Source: CAD feature listing. Evaluate the final solid. Frame: model axes, mm. A direction names the side the tool comes from. Coordinates: 2 decimals unless noted, no trailing zeros. Order: outer loops, then holes, each group sorted by start corner. A loop starts at its lowest first (then second) coordinate and runs counter-clockwise, first axis right, second up.
Autodesk Inventor part; units mm, degrees
ref_plane "YZ Plane" through (0, 0, 0) normal (1, 0, 0) x (0, 1, 0)
ref_plane "XZ Plane" through (0, 0, 0) normal (0, 1, 0) x (-1, 0, 0)
ref_plane "XY Plane" through (0, 0, 0) normal (0, 0, 1) x (1, 0, 0)
sketch "Sketch1" plane through (0, 0, 0) normal (0, 1, 0) x (-1, 0, 0)
  line L0 (0, 0) -> (-38.1, 0)
  line L1 (-38.1, 0) -> (-38.1, -38.1)
  line L2 (-38.1, -38.1) -> (0, -38.1)
  line L3 (0, -38.1) -> (0, 0)
  dimension "d0" = 38.1
  dimension "d1" = 38.1
extrude "Extrusion1" add sketch "Sketch1" along normal blind 25.4
fillet "Fillet1" radius 19.05 1 edges at (0, 12.7, 0)
sketch "Sketch2" plane through (0, 25.4, 0) normal (0, 1, 0) x (1, 0, 0)
  arc A0 (0, 19.05) -> (19.05, 0) centre (19.05, 19.05) ccw
  line L0 (0, 38.1) -> (0, 19.05)
  line L1 (38.1, 38.1) -> (0, 38.1)
  line L2 (38.1, 0) -> (38.1, 38.1)
  line L3 (19.05, 0) -> (38.1, 0)
  arc A1 (-2.8591, 19.05) -> (19.05, -2.8591) centre (19.05, 19.05) ccw
  line L4 (-2.8591, 19.05) -> (-2.8591, 40.9591)
  line L5 (-2.8591, 40.9591) -> (40.9591, 40.9591)
  line L6 (40.9591, 40.9591) -> (40.9591, -2.8591)
  line L7 (40.9591, -2.8591) -> (19.05, -2.8591)
  line L8 (0, 38.1) -> (0, 40.9591)
  line L9 (38.1, 0) -> (40.9591, 0)
  point P0 (0, 0)
extrude "Extrusion2" add sketch "Sketch2" along normal blind 44.45 contours A0 L3 L9 L6 L7 A1 L4 L5 L8 L0
sketch "Sketch3" plane through (0, 25.4, 0) normal (0, 1, 0) x (1, 0, 0)
  arc A0 (0, 19.05) -> (19.05, 0) centre (19.05, 19.05) ccw
  line L0 (19.05, 0) -> (38.1, 0)
  line L1 (38.1, 0) -> (38.1, 38.1)
  line L2 (38.1, 38.1) -> (0, 38.1)
  line L3 (0, 38.1) -> (0, 19.05)
  point P0 (0, 0)
extrude "Extrusion3" cut sketch "Sketch3" against normal blind 44.45
sketch "Sketch4" plane through (0, 69.85, 0) normal (0, 1, 0) x (1, 0, 0)
  arc A0 (0, 19.05) -> (19.05, 0) centre (19.05, 19.05) ccw
  line L0 (0, 19.05) -> (0, 40.9591)
  line L1 (0, 40.9591) -> (-2.8591, 40.9591)
  line L2 (-2.8591, 40.9591) -> (-2.8591, 19.05)
  arc A1 (-2.8591, 19.05) -> (19.05, -2.8591) centre (19.05, 19.05) ccw
  line L3 (19.05, -2.8591) -> (40.9591, -2.8591)
  line L4 (40.9591, -2.8591) -> (40.9591, 0)
  line L5 (40.9591, 0) -> (19.05, 0)
  point P0 (0, 0)
extrude "Extrusion4" add sketch "Sketch4" along normal blind 660.4
properties part number "Cart_Side_Beam"
1. Section query B-B on z = -26.5. Return loops of the section in (x, y), plus the area to 3 significant figures.
Findings:
outline: (-2.86, 25.4) - (0, 25.4) - (0, 730.25) - (-2.86, 730.25) - close
area: 2,020 mm2
2. Access query for faces 1 (the face through (30, 373, 0)), 2 (the face through (3.73, 372.89, -3.39)). Directions: +Z, -Z, +X, -X, +Y, -Y. A direction counts if a zero-diameter tool reaches every point of the face in a straight line with its end or side. Return the directions, or none.
Findings:
face 1: -Z, +X, +Y, -Y
face 2: +Z, -X, +Y, -Y
3. Section query A-A on y = 387.5. Return loops of the section in (x, z).
Findings:
outline: (-2.86, -40.96) - (0, -40.96) - (0, -19.05) arc R19.05 cw to (19.05, 0) - (40.96, 0) - (40.96, 2.86) - (19.05, 2.86) arc R21.91 ccw to (-2.86, -19.05) - close
4. Pin query (flat end, axial travel): P1, Ø17.5, axis at y = 315, z = -31.5, coming from the +X side; P2, Ø1.5, axis at y = 376.5, z = -4.5, coming from the -X side; P3, Ø1, axis at y = 514, z = -16.5, coming from the -X side. Return the tip coordinate at first contact, or that it passes through.
Findings:
P1: stops at x = 0
P2: stops at x = 2.03
P3: stops at x = -2.76
5. Section query C-C on x = 6. Return loops of the section in (y, z).
Findings:
outline: (25.4, -5.17) - (730.25, -5.17) - (730.25, -1.45) - (25.4, -1.45) - close
6. Ray query, line 1 (X direction, y = 62, z = -21.5); line 2 (Z direction, x = 31, y = 559); line 3 (X direction, y = 120, z = -18). Return the intervals inside material, ascending.
Findings:
line 1: x = -2.86 to 0
line 2: z = 0 to 2.86
line 3: x = -2.83 to 0.03
